from build123d import *

# Parameters (mm, degrees)
F0_R     = 368.3
F1_DEPTH = 25.4
F0_R_2   = 381
F2_DEPTH = 914.4
F3_R     = 393.7
F3_R_2   = 381
F4_DEPTH = 12.7
F5_R     = 393.7
F5_R_2   = 381
F6_DEPTH = 12.7


with BuildPart() as f1:
    # F0 (on Top) → F1 (new body)
    with BuildSketch(Plane.XY):
        Circle(F0_R)
    extrude(amount=F1_DEPTH)

    # F0 (on Top) → F2 (join)
    with BuildSketch(Plane.XY):
        Circle(F0_R_2)
        Circle(F0_R, mode=Mode.SUBTRACT)
    extrude(amount=F2_DEPTH)

    # F3 (on face) → F4 (join)
    with BuildSketch(Plane(origin=(0, 0, 0), x_dir=(1, 0, 0), z_dir=(0, 0, -1))):
        Circle(F3_R)
        Circle(F3_R_2, mode=Mode.SUBTRACT)
    extrude(amount=-F4_DEPTH)

    # F5 (on face) → F6 (join)
    with BuildSketch(Plane.XY.offset(914.4)):
        Circle(F5_R)
        Circle(F5_R_2, mode=Mode.SUBTRACT)
    extrude(amount=-F6_DEPTH)


solid = f1.part
Check sheet for the modelled part. Datum: model origin and axes. Units: mm. A direction names the side the tool comes from. Give positions to 0.01 mm unless a question says otherwise; leave off trailing zeros. Loops run counter-clockwise (first coordinate to the right, second up) from the corner with the lowest first, then second, coordinate; pieces in that order, holes last. Notation, with made-up numbers: M 58,-23 L 65,-23 A32 ccw 65,5 Z; hole C 78,14.25 d6. An arc over 180 degrees is marked long. Return JSON: item names as keys, results as strings. Group by question number.
1. Go/stop test with flat-tipped pins: pin 1 (5 mm diameter, centred on x = -2.5, y = 155, fed in from -Z); pin 2 (1.5 mm diameter, centred on y = 158.5, z = 474.5, fed in from +X); pin 3 (4 mm diameter, centred on x = -278.5, z = 372, fed in from +Y); pin 4 (2 mm diameter, centred on y = 83, z = 473.5, fed in from -X). Record where each tip stops, or that it passes through.
2. Mould release check, pull along X, two halves, no side actions. Record for faces 1 (the cylindrical face through (-292.27, -224.105, 463.677)), 2 (the flat face through (-206, 323, 901.7)), 3 (the cylindrical face through (375.52, -118.26, 6.26)): released by +X, released by -X, zero draft, split by the parting line, or undercut.
3. Tool access check on faces 4 (the cylindrical face through (-302.35, -231.83, 450.98)), 5 (the flat face through (-5, 5, 25.4)), 6 (the flat face through (261, -261, 914.4)). Record the directions out of +Z, -Z, +X, -X, +Y, -Y that give a thin tool (end or side, any length) a straight path to the whole face; none if there is none.
4. Cross-section at C-C on z = 147. Record the boundary of the cut face in (x, y).
5. Cross-section at A-A on x = 0. Record the boundary of the cut face in (y, z).
6. Thickness scan on L1, parallel to Y at x = 0, z = 308; L2, parallel to Z at x = 246.5, y = -159; L3, parallel to Y at x = 116, z = 81. Record the ranges inside material, lowest first.
Return value:
{
 "1": {"pin 1": "z = 0", "pin 2": "x = 346.81", "pin 3": "y = 262.12", "pin 4": "x = -372.07"},
 "2": {"face 1": "undercut", "face 2": "zero draft", "face 3": "split by the parting line"},
 "3": {"face 4": "none", "face 5": "+Z", "face 6": "+Z, +X, -X, +Y, -Y"},
 "4": {"outline": "C 0,0 d762; hole C 0,0 d736.6"},
 "5": {"outline": "M -393.7,0 L 393.7,0 L 393.7,12.7 L 381,12.7 L 381,901.7 L 393.7,901.7 L 393.7,914.4 L 368.3,914.4 L 368.3,25.4 L -368.3,25.4 L -368.3,914.4 L -393.7,914.4 L -393.7,901.7 L -381,901.7 L -381,12.7 L -393.7,12.7 Z"},
 "6": {"L1": "-381 to -368.3, 368.3 to 381", "L2": "0 to 25.4", "L3": "-362.91 to -349.56, 349.56 to 362.91"}
}
